```python
from build123d import *

# Parameters (mm, degrees)
SKETCH_1_W            = 24.4475
SKETCH_1_H            = 33.02
SKETCH_1_R            = 0.44958
SKETCH_1_R_2          = 0.55118
SKETCH_1_R_3          = 0.59944
SKETCH_1_R_4          = 0.50038
SKETCH_1_R_5          = 0.4445
EXTRUDE_1_DEPTH       = 1.5
EXTRUDE_2_OUTLINE_W   = 1.6002
EXTRUDE_2_OUTLINE_H   = 1.40208
EXTRUDE_2_OUTLINE_H_2 = 1.39954
EXTRUDE_2_DEPTH       = 0.1


# Read off the part's stored shape, not the designer's step: Бобышка-Вытянуть2
with BuildPart() as part:
    # Эскиз1 → Бобышка-Вытянуть1 (new body)
    with BuildSketch(Plane.XY):
        with Locations((12.22375, 16.51)):
            Rectangle(SKETCH_1_W, SKETCH_1_H)
        with Locations((19.685, 21.59)):
            Circle(SKETCH_1_R, mode=Mode.SUBTRACT)
        with Locations((19.685, 24.13)):
            Circle(SKETCH_1_R, mode=Mode.SUBTRACT)
        with Locations((12.065, 24.13)):
            Circle(SKETCH_1_R, mode=Mode.SUBTRACT)
        with Locations((12.065, 21.59)):
            Circle(SKETCH_1_R, mode=Mode.SUBTRACT)
        with Locations((14.605, 15.875)):
            Circle(SKETCH_1_R_2, mode=Mode.SUBTRACT)
        with Locations((14.605, 18.415)):
            Circle(SKETCH_1_R_3, mode=Mode.SUBTRACT)
        with Locations((14.605, 2.54)):
            Circle(SKETCH_1_R_3, mode=Mode.SUBTRACT)
        with Locations((14.605, 5.08)):
            Circle(SKETCH_1_R_3, mode=Mode.SUBTRACT)
        with Locations((9.906, 27.305)):
            Circle(SKETCH_1_R_4, mode=Mode.SUBTRACT)
        with Locations((20.955, 27.305)):
            Circle(SKETCH_1_R_4, mode=Mode.SUBTRACT)
        with Locations((8.89, 29.845)):
            Circle(SKETCH_1_R_5, mode=Mode.SUBTRACT)
        with Locations((6.35, 29.845)):
            Circle(SKETCH_1_R_5, mode=Mode.SUBTRACT)
    extrude(amount=EXTRUDE_1_DEPTH)

    # Бобышка-Вытянуть2 outline → Бобышка-Вытянуть2 (add)
    with BuildSketch(Plane.XY.offset(1.5)):
        with Locations((3.429, 1.905)):
            Rectangle(EXTRUDE_2_OUTLINE_W, EXTRUDE_2_OUTLINE_H)
        with Locations((3.429, 6.40461)):
            Rectangle(EXTRUDE_2_OUTLINE_W, EXTRUDE_2_OUTLINE_H_2)
        with Locations((11.43, 1.905)):
            Rectangle(EXTRUDE_2_OUTLINE_W, EXTRUDE_2_OUTLINE_H)
        with Locations((11.43, 6.40461)):
            Rectangle(EXTRUDE_2_OUTLINE_W, EXTRUDE_2_OUTLINE_H_2)
    extrude(amount=EXTRUDE_2_DEPTH)


solid = part.part
```
The model under review builds one solid part; all positions refer to its coordinate system, in mm. Give positions to 0.01 mm unless a question says otherwise; leave off trailing zeros. Order: outer loops, then holes, each group sorted by start corner. A loop starts at its lowest first (then second) coordinate and runs counter-clockwise, first axis right, second up. Notation, with made-up numbers: (21.25, 85) - (54.25, 85) arc R3 cw to (54.25, 90) - close; hole circle Ø8 at (75.5, 47.5). An arc over 180 degrees is marked (long way). Use CSV: the item, a comma, the result in double quotes. Start each with the question number.
Q1. We need section D-D, the plane x = 18.5. Write out the cut boundary in (y, z), and give its area (3 significant figures).
Q2. We need section C-C, the plane y = 5.08. Write out the cut boundary in (x, z).
Q3. We need section B-B, the plane y = 21.59. Write out the cut boundary in (x, z).
Q4. We need section A-A, the plane x = 6.35. Write out the cut boundary in (y, z).
Q5. The part is to be moulded in two halves that separate along X. For faces 1 (the cylindrical face through (19.927, 21.969, 0.74)), 2 (the cylindrical face through (14.93, 18.92, 0.74)), 3 (the flat face through (0, 16, 1)), 4 (the flat face through (12, 17, 0)), say which applies: +X half, -X half, draft (parallel to the pull), parting line (faces both ways), or undercut.
Q6. To check wall thickness, follow line 1 along X through (y, z) = (24.13, 1.1); line 2 along Y through (x, z) = (6.35, 0.9); line 3 along Y through (x, z) = (20, 1.05). State the ranges of each line that lie inside material, in increasing order. Write a range as [from, to].
Q7. Clearance check with flat-ended pins moving along their axes: pin 1 Ø1.2 at (x, y) = (9.906, 27.305) entering from -Z; pin 2 Ø1.6 at (x, y) = (20.955, 27.305) entering from +Z. State where each tip first meets the part, or that it passes through.
Outcome:
1,outline,"(0, 0) - (33.02, 0) - (33.02, 1.5) - (0, 1.5) - close"
1,area,"49.5 mm^2"
2,outline,"(0, 0) - (14.01, 0) - (14.01, 1.5) - (0, 1.5) - close; (15.2, 0) - (24.45, 0) - (24.45, 1.5) - (15.2, 1.5) - close"
3,outline,"(0, 0) - (11.62, 0) - (11.62, 1.5) - (0, 1.5) - close; (12.51, 0) - (19.24, 0) - (19.24, 1.5) - (12.51, 1.5) - close; (20.13, 0) - (24.45, 0) - (24.45, 1.5) - (20.13, 1.5) - close"
4,outline,"(0, 0) - (29.4, 0) - (29.4, 1.5) - (0, 1.5) - close; (30.29, 0) - (33.02, 0) - (33.02, 1.5) - (30.29, 1.5) - close"
5,face 1,"undercut"
5,face 2,"undercut"
5,face 3,"-X half"
5,face 4,"draft"
6,line 1,"x = [0, 11.62], [12.51, 19.24], [20.13, 24.45]"
6,line 2,"y = [0, 29.4], [30.29, 33.02]"
6,line 3,"y = [0, 21.27], [21.91, 23.81], [24.45, 33.02]"
7,pin 1,"stops at z = 0"
7,pin 2,"stops at z = 1.5"
